from build123d import *

# Parameters (mm, degrees)
F0_W     = 50
F0_H     = 10
F0_R     = 2.6
F1_DEPTH = 5
F2_W     = 10
F2_H     = 3
F3_DEPTH = 10
F4_W     = 7
F4_H     = 3
F5_DEPTH = 8
F7_DEPTH = 10


with BuildPart() as f1:
    # F0 (on Top) → F1 (new body)
    with BuildSketch(Plane.XY):
        with Locations((20, 0)):
            Rectangle(F0_W, F0_H)
        Circle(F0_R, mode=Mode.SUBTRACT)
        with Locations((40, 0)):
            Circle(F0_R, mode=Mode.SUBTRACT)
    extrude(amount=F1_DEPTH)

    # F2 (on face) → F3 (join)
    with BuildSketch(Plane(origin=(0, 5, 0), x_dir=(-1, 0, 0), z_dir=(0, 1, 0))):
        Polygon((-35, 5), (-5, 5), (-14, 24), (-20, 24), (-26, 24), align=None)
        with Locations((-20, 17.5)):
            Rectangle(F2_W, F2_H, mode=Mode.SUBTRACT)
    extrude(amount=-F3_DEPTH)

    # F4 (on face) → F5 (cut)
    with BuildSketch(Plane.XY.offset(24)):
        with Locations((20, -1.5)):
            Rectangle(F4_W, F4_H)
    extrude(amount=-F5_DEPTH, mode=Mode.SUBTRACT)

    # F6 (on face) → F7 (cut, through all)
    with BuildSketch(Plane(origin=(0, 5, 0), x_dir=(-1, 0, 0), z_dir=(0, 1, 0))):
        Polygon((-15, 13), (-25, 13), (-28.789474, 5), (-11.210526, 5), align=None)
    extrude(amount=-F7_DEPTH, mode=Mode.SUBTRACT)


solid = f1.part
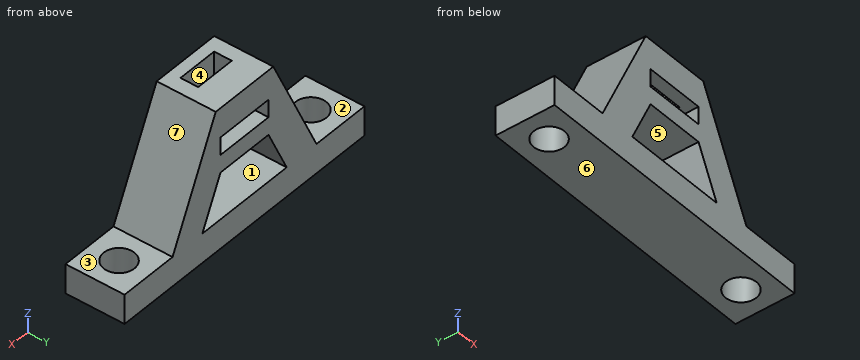
Source: CAD feature listing. Evaluate the final solid. Frame: model axes, mm. Face numbers are marked on the shaded views. A direction names the side the tool comes from. Round coordinates to 2 decimals unless told otherwise and drop trailing zeros. Loops run counter-clockwise (first coordinate to the right, second up) from the corner with the lowest first, then second, coordinate; pieces in that order, holes last. Notation, with made-up numbers: M 59.25,55 L 69.25,55 A29 cw 69.25,75 Z; hole C -5,40 d1. An arc over 180 degrees is marked long. Return JSON: item names as keys, results as strings. Group by question number.
1. Reachability of the marked faces 1, 2 and 3 from +Z, -Z, +X, -X, +Y, -Y: full face, straight path, thin tool, end or side. Return the list, or none.
2. Material intervals for line 1 along Z through (x, y) = (15.5, -3.25); line 2 along X through (y, z) = (0.5, 3); line 3 along Z through (x, y) = (41, 3.25), sorted ascending. Write a range as from..to.
3. Pin query (flat end, axial travel): pin 1 (2 mm diameter, centred on y = -2.5, z = 19, fed in from +X); pin 2 (5 mm diameter, centred on y = 3, z = 17.5, fed in from +X); pin 3 (1.5 mm diameter, centred on y = 2, z = 18, fed in from +X). Return the tip coordinate at first contact, or that it passes through.
4. Section query D-D on y = -0.5. Output: boundary loops of the cut face in (x, z), and give its area (3 significant figures).
5. Mould query, pull axis X, two halves, no side actions, for the marked faces 4, 5, 6 and 7. Classes: released by +X, released by -X, zero draft, split by the parting line, or undercut.
6. Section query A-A on x = 20.5. Output: boundary loops of the cut face in (y, z), and give its area (3 significant figures).
7. Section query B-B on y = 1.5. Output: boundary loops of the cut face in (x, z).
8. Section query C-C on x = 40. Output: boundary loops of the cut face in (y, z), and give its area (3 significant figures).
Checks:
{
 "1": {"face 1": "+Y, -Y", "face 2": "+Z, -X, +Y, -Y", "face 3": "+Z, +X, +Y, -Y"},
 "2": {"line 1": "z = 0..5, 13..16, 19..24", "line 2": "x = -5..-2.55, 2.55..37.45, 42.55..45", "line 3": "z = 0..5"},
 "3": {"pin 1": "stops at x = 28.84", "pin 2": "stops at x = 30.26", "pin 3": "stops at x = 29.2"},
 "4": {"outline": "M -5,0 L -2.55,0 L -2.55,5 L -5,5 Z; M 2.55,0 L 37.45,0 L 37.45,5 L 35,5 L 26,24 L 23.5,24 L 23.5,19 L 25,19 L 25,16 L 15,16 L 15,19 L 16.5,19 L 16.5,24 L 14,24 L 5,5 L 2.55,5 Z; M 42.55,0 L 45,0 L 45,5 L 42.55,5 Z; hole M 11.21,5 L 28.79,5 L 25,13 L 15,13 Z", "area": "423 mm²"},
 "5": {"face 4": "undercut", "face 5": "undercut", "face 6": "zero draft", "face 7": "released by +X"},
 "6": {"outline": "M -5,0 L 5,0 L 5,5 L -5,5 Z; M -5,13 L 5,13 L 5,16 L -5,16 Z; M -5,19 L -3,19 L -3,24 L -5,24 Z; M 0,19 L 5,19 L 5,24 L 0,24 Z", "area": "115 mm²"},
 "7": {"outline": "M -5,0 L -2.12,0 L -2.12,5 L -5,5 Z; M 2.12,0 L 37.88,0 L 37.88,5 L 35,5 L 26,24 L 14,24 L 5,5 L 2.12,5 Z; M 42.12,0 L 45,0 L 45,5 L 42.12,5 Z; hole M 11.21,5 L 28.79,5 L 25,13 L 15,13 Z; hole M 15,16 L 25,16 L 25,19 L 15,19 Z"},
 "8": {"outline": "M -5,0 L -2.6,0 L -2.6,5 L -5,5 Z; M 2.6,0 L 5,0 L 5,5 L 2.6,5 Z", "area": "24.0 mm²"}
}
